The listing builds one solid part. Answer for the finished solid, in the listing's coordinates (mm). A direction names the side the tool comes from. Round coordinates to 2 decimals unless told otherwise and drop trailing zeros. Order: outer loops, then holes, each group sorted by start corner. A loop starts at its lowest first (then second) coordinate and runs counter-clockwise, first axis right, second up. Notation, with made-up numbers: (80.5, -18.5) - (97.5, -18.5) arc R33 cw to (97.5, 10.5) - close; hole circle Ø8 at (-38, 89). An arc over 180 degrees is marked (long way). Write item = value, one per line.
from build123d import *

# Parameters (mm, degrees)
ESQUISSE2_R                  = 4
ENL_V_MAT_EXTRU_1_DEPTH      = 20.75
ENL_V_MAT_EXTRU_1_DEPTH_BACK = 20.75
CONG_2_R                     = 2


with BuildPart() as part:
    # Esquisse1 → Base-Révolution (revolve)
    with BuildSketch(Plane.XY):
        Polygon((-24, 10), (-24, 19.75), (-7.2, 19.75), (-7.2, 16.75), (-3, 16.75), (-3, 19.75), (-1.5, 19.75), (1, 17.25), (1, 10), (-0.4, 10), (-0.4, 11.5), (-3, 11.5), (-3, 10), align=None)
    revolve(axis=Axis((-92, 0, 0), (1, 0, 0)))

    # Esquisse2 → Enlèv. mat.-Extru.1 (cut, two sides)
    with BuildSketch(Plane.XY) as enl_v_mat_extru_1_sk:
        with Locations((-15, 0)):
            Circle(ESQUISSE2_R)
    extrude(amount=ENL_V_MAT_EXTRU_1_DEPTH, mode=Mode.SUBTRACT)
    extrude(enl_v_mat_extru_1_sk.sketch, amount=-ENL_V_MAT_EXTRU_1_DEPTH_BACK, mode=Mode.SUBTRACT)

    # Congé2
    cong_2_edges = [part.edges().sort_by_distance(p)[0] for p in [
        (-24, -19.75, 0),
    ]]
    fillet(cong_2_edges, radius=CONG_2_R)


solid = part.part
Q1. Section D-D on y = 0 is taken. Count the separate pieces of the cut face and the enclosed holes in it, then the cut area to 3 significant figures.
Model answer:
separate_pieces = 4
enclosed_holes = 0
area = 291 mm^2
Q2. Section A-A on z = 0 is taken. Determine the outline of the cut face in (x, y).
Model answer:
outline = (-24, -17.75) arc R2 ccw to (-22, -19.75) - (-7.2, -19.75) - (-7.2, -16.75) - (-3, -16.75) - (-3, -19.75) - (-1.5, -19.75) - (1, -17.25) - (1, -10) - (-0.4, -10) - (-0.4, -11.5) - (-3, -11.5) - (-3, -10) - (-24, -10) - close; (-24, 10) - (-3, 10) - (-3, 11.5) - (-0.4, 11.5) - (-0.4, 10) - (1, 10) - (1, 17.25) - (-1.5, 19.75) - (-3, 19.75) - (-3, 16.75) - (-7.2, 16.75) - (-7.2, 19.75) - (-22, 19.75) arc R2 ccw to (-24, 17.75) - close
Q3. Find the intervals of material crossed by line 1 (X direction, y = 0, z = -15); line 2 (X direction, y = 0, z = -11); line 3 (X direction, y = 14.5, z = 11.5), in increasing order. Write a range as from..to.
Model answer:
line_1 = -24..-19, -11..1
line_2 = -24..-19, -11..-3, -0.4..1
line_3 = -23.85..-7.2, -3..-0.26
Q4. Section C-C on x = -20.5 is taken. Determine the outline of the cut face in (y, z), then the cut area to 3 significant figures.
Model answer:
outline = circle Ø39.5 at (0, 0); hole circle Ø20 at (0, 0)
area = 911 mm^2
Q5. Section B-B on x = -15 is taken. Determine the outline of the cut face in (y, z), then the cut area to 3 significant figures.
Model answer:
outline = (-4, -19.34) - (-4, -9.17) arc R10 cw to (-4, 9.17) - (-4, 19.34) arc R19.75 ccw to start; (4, -19.34) arc R19.75 ccw to (4, 19.34) - (4, 9.17) arc R10 cw to (4, -9.17) - close
area = 753 mm^2
Q6. Flat-ended cylindrical pins translate along their axes: P1, Ø10, axis at x = -20.5, y = -10, coming from the +Z side; P2, Ø1, axis at x = -21.5, z = -6.5, coming from the +Y side; P3, Ø1, axis at x = -4.5, z = 7, coming from the -Y side. Find the tip coordinate at first contact, or state that the pin passes through.
Model answer:
P1 = 19.11
P2 = 18.82
P3 = -15.44
Q7. Determine the mould class of faces 3 (the face through (-0.4, 9, 5)), 4 (the face through (1, 7.4, -7.4)), 5 (the face through (0.29, -2.17, -9.76)) for opening direction X: released by +X, released by -X, zero draft, split by the parting line, or undercut.
Model answer:
face_3 = undercut
face_4 = released by +X
face_5 = zero draft
Q8. For faces 1 (the face through (-24, -8, -8)), 2 (the face through (-3, -9, 5)), determine the directions among +Z, -Z, +X, -X, +Y, -Y from which every point of the face is accessible in a straight line to the end or side of a thin tool.
Model answer:
face_1 = +Z, -Z, -X, +Y, -Y
face_2 = none
